Design review of the part built by this model. Coordinates are the model's own, in mm. A direction names the side the tool comes from. Coordinates: 2 decimals unless noted, no trailing zeros. Order: outer loops, then holes, each group sorted by start corner. A loop starts at its lowest first (then second) coordinate and runs counter-clockwise, first axis right, second up. Notation, with made-up numbers: (-19.5, 19) -> (12.5, 19) arc R5 ccw to (12.5, 27) -> close; hole circle Ø1 at (21, 52.25). An arc over 180 degrees is marked (long way). Use a Markdown table: item, result. Add a question column.
Q1. Add section A-A (y = 2). State the section outline as (x, z) points, then the cut area to 3 significant figures.
Q2. Add section B-B (z = 17.5). State the section outline as (x, y) points, then the cut area to 3 significant figures.
Q3. Machinability: for faces 4 (the face through (5.959, 6.738, 24.061)), 5 (the face through (6.6, 7.7, 24.2)), 6 (the face through (3, 8, 42)), which of the approach directions +Z, -Z, +X, -X, +Y, -Y give a long, thin tool a straight path to every point of the face, cutting with its end or side? Answer none if there is none.
Q4. The part is to be moulded in two halves that separate along X. For faces 1 (the face through (5, 9, 36)), 2 (the face through (6.55, 5.16, 38.77)), 3 (the face through (4, 0, 5)), say which applies: pulls with the +X half, pulls with the -X half, needs draft (parallel to the pull), parting line crosses it, or undercut.
Q5. Wall thickness on probe 1 along X at (y, z) = (1.3, 3); probe 2 along Z at (x, y) = (2.75, 12.5); probe 3 along Z at (x, y) = (3.5, 5.5): over which ranges is each line inside the solid? List them lowest first.
Q6. Add section C-C (z = 3). State the section outline as (x, y) points, then the cut area to 3 significant figures.
Q7. Add section D-D (z = 10.5). State the section outline as (x, y) points.
Q8. Insertion check: pin 1 (1.8 mm diameter, centred on x = 5.5, z = 45, fed in from +Y); pin 2 (2 mm diameter, centred on x = 4.5, y = 8.5, fed in from +Z); pin 3 (2 mm diameter, centred on x = 5.5, y = 9, fed in from -Z). Each pin has a flat end and moves straight along its axis. Give the tip position at first contact, or say it passes through.
from build123d import *

# Parameters (mm, degrees)
SKETCH_1_W          = 8
SKETCH_1_H          = 15
EXTRUDE_1_DEPTH     = 48
SKETCH_2_W          = 8
SKETCH_2_H          = 6
CUT_EXTRUDE_1_DEPTH = 12
SKETCH_4_W          = 8
SKETCH_4_H          = 32
CUT_EXTRUDE_3_DEPTH = 4
SKETCH_5_R          = 1.6
CUT_EXTRUDE_4_DEPTH = 3
FILLET_1_R          = 2
CUT_EXTRUDE_5_DEPTH = 32
SKETCH_6_W          = 30
SKETCH_6_H          = 8
CUT_EXTRUDE_6_DEPTH = 1
CHAMFER_1_SIZE      = 7
FILLET_2_R          = 0.8
CUT_EXTRUDE_7_DEPTH = 10
CUT_EXTRUDE_8_DEPTH = 0.2


with BuildPart() as part:
    # 草图1 → 凸台-拉伸1 (new body)
    with BuildSketch(Plane.XY):
        with Locations((4, 7.5)):
            Rectangle(SKETCH_1_W, SKETCH_1_H)
    extrude(amount=EXTRUDE_1_DEPTH)

    # 草图2 → 切除-拉伸1 (cut)
    with BuildSketch(Plane(origin=(0, 15, 0), x_dir=(1, 0, 0), z_dir=(0, 1, 0))):
        with Locations((4, -3)):
            Rectangle(SKETCH_2_W, SKETCH_2_H)
        with Locations((4, -45)):
            Rectangle(SKETCH_2_W, SKETCH_2_H)
    extrude(amount=-CUT_EXTRUDE_1_DEPTH, mode=Mode.SUBTRACT)

    # 草图4 → 切除-拉伸3 (cut)
    with BuildSketch(Plane.XZ):
        with Locations((4, 24)):
            Rectangle(SKETCH_4_W, SKETCH_4_H)
    extrude(amount=-CUT_EXTRUDE_3_DEPTH, mode=Mode.SUBTRACT)

    # 草图5 → 切除-拉伸4 (cut)
    with BuildSketch(Plane(origin=(0, 3, 0), x_dir=(1, 0, 0), z_dir=(0, 1, 0))):
        with Locations(Location((4, -3, 0), (0, 0, 270))):
            Circle(SKETCH_5_R)
        with Locations(Location((4, -45, 0), (0, 0, 270))):
            Circle(SKETCH_5_R)
    extrude(amount=-CUT_EXTRUDE_4_DEPTH, mode=Mode.SUBTRACT)

    # 圆角1
    fillet_1_edges = [part.edges().sort_by_distance(p)[0] for p in [
        (8, 1.5, 48),
        (0, 1.5, 0),
        (0, 1.5, 48),
        (8, 1.5, 0),
    ]]
    fillet(fillet_1_edges, radius=FILLET_1_R)

    # 草图3 → 切除-拉伸5 (cut)
    with BuildSketch(Plane.XY.offset(40)):
        Polygon((0, 4), (7, 4), (0, 11), align=None)
    extrude(amount=-CUT_EXTRUDE_5_DEPTH, mode=Mode.SUBTRACT)

    # 草图6 → 切除-拉伸6 (cut)
    with BuildSketch(Plane(origin=(5.5, 5.5, 0), x_dir=(0, 0, 1), z_dir=(-0.7071067811865474, -0.7071067811865477, 0))):
        with Locations((24, 2.778174593)):
            Rectangle(SKETCH_6_W, SKETCH_6_H)
    extrude(amount=-CUT_EXTRUDE_6_DEPTH, mode=Mode.SUBTRACT)

    # 倒角1
    chamfer_1_edges = [part.edges().sort_by_distance(p)[0] for p in [
        (8, 15, 24),
    ]]
    chamfer(chamfer_1_edges, length=CHAMFER_1_SIZE)

    # 圆角2
    fillet_2_edges = [part.edges().sort_by_distance(p)[0] for p in [
        (6.717514421, 4.98959236, 9),
        (1.060660172, 10.646446609, 9),
        (1.060660172, 10.646446609, 39),
        (6.717514421, 4.98959236, 39),
    ]]
    fillet(fillet_2_edges, radius=FILLET_2_R)

    # 草图7 → 切除-拉伸7 (cut)
    with BuildSketch(Plane(origin=(6.207106781, 6.207106781, 0), x_dir=(0, 0, 1), z_dir=(-0.7071067811865475, -0.7071067811865477, 0))):
        with BuildLine():
            Line((13.2, 4.778174593), (34.8, 4.778174593))
            ThreePointArc((34.8, 4.778174593), (35.648528137, 4.42670273), (36, 3.578174593))
            Line((36, 3.578174593), (36, 1.978174593))
            ThreePointArc((36, 1.978174593), (35.648528137, 1.129646456), (34.8, 0.778174593))
            Line((34.8, 0.778174593), (13.2, 0.778174593))
            ThreePointArc((13.2, 0.778174593), (12.351471863, 1.129646456), (12, 1.978174593))
            Line((12, 1.978174593), (12, 3.578174593))
            ThreePointArc((12, 3.578174593), (12.351471863, 4.42670273), (13.2, 4.778174593))
        make_face()
    extrude(amount=-CUT_EXTRUDE_7_DEPTH, mode=Mode.SUBTRACT)

    # 草图8 → 切除-拉伸8 (cut)
    with BuildSketch(Plane(origin=(6.207106781, 6.207106781, 0), x_dir=(0, 0, 1), z_dir=(-0.7071067811865475, -0.7071067811865477, 0))):
        with BuildLine():
            Line((12, 5.528174593), (36, 5.528174593))
            ThreePointArc((36, 5.528174593), (36.707106781, 5.235281374), (37, 4.528174593))
            Line((37, 4.528174593), (37, 1.028174593))
            ThreePointArc((37, 1.028174593), (36.707106781, 0.321067812), (36, 0.028174593))
            Line((36, 0.028174593), (12, 0.028174593))
            ThreePointArc((12, 0.028174593), (11.292893219, 0.321067812), (11, 1.028174593))
            Line((11, 1.028174593), (11, 4.528174593))
            ThreePointArc((11, 4.528174593), (11.292893219, 5.235281374), (12, 5.528174593))
        make_face()
    extrude(amount=-CUT_EXTRUDE_8_DEPTH, mode=Mode.SUBTRACT)


solid = part.part
Established:
| question | item | result |
|---|---|---|
| 1 | outline | (0, 2) arc R2 ccw to (2, 0) -> (6, 0) arc R2 ccw to (8, 2) -> (8, 8) -> (0, 8) -> close; (0, 40) -> (8, 40) -> (8, 46) arc R2 ccw to (6, 48) -> (2, 48) arc R2 ccw to (0, 46) -> close; hole circle Ø3.2 at (4, 3); hole circle Ø3.2 at (4, 45) |
| 1 | area | 108 mm^2 |
| 2 | outline | (0, 11) -> (0.71, 10.29) -> (1.41, 11) -> (2.3, 10.12) -> (2.44, 10.26) -> (2.97, 9.73) -> (4.62, 11.38) -> (1, 15) -> (0, 15) -> close; (5.8, 6.9) -> (6.33, 6.37) -> (6.19, 6.23) -> (7.07, 5.34) -> (6.36, 4.64) -> (7, 4) -> (8, 4) -> (8, 8) -> (7.45, 8.55) -> close |
| 2 | area | 20.6 mm^2 |
| 3 | face 4 | none |
| 3 | face 5 | -X, +Y |
| 3 | face 6 | +Z, +X, -X, +Y |
| 4 | face 1 | undercut |
| 4 | face 2 | pulls with the -X half |
| 4 | face 3 | needs draft |
| 5 | probe 1 | 0 to 2.4, 5.6 to 8 |
| 5 | probe 2 | 6 to 42 |
| 5 | probe 3 | 6 to 8, 40 to 42 |
| 6 | outline | (0, 0) -> (2.4, 0) -> (2.4, 3) -> (0, 3) -> close; (5.6, 0) -> (8, 0) -> (8, 3) -> (5.6, 3) -> close |
| 6 | area | 14.4 mm^2 |
| 7 | outline | (0, 11) -> (0.71, 10.29) -> (1.41, 11) -> (7.07, 5.34) -> (6.36, 4.64) -> (7, 4) -> (8, 4) -> (8, 8) -> (1, 15) -> (0, 15) -> close |
| 8 | pin 1 | y = 3 |
| 8 | pin 2 | z = 42 |
| 8 | pin 3 | z = 6 |
